Model file for the job. Use its own axes, mm. Face numbers are marked on the shaded views. A direction names the side the tool comes from. Give positions to 0.01 mm unless a question says otherwise; leave off trailing zeros. Order: outer loops, then holes, each group sorted by start corner. A loop starts at its lowest first (then second) coordinate and runs counter-clockwise, first axis right, second up. Notation, with made-up numbers: (-24.75, 48.5) - (0.25, 48.5) arc R14 cw to (0.25, 62.5) - close; hole circle Ø4 at (13.5, 47.5). An arc over 180 degrees is marked (long way). Return JSON: item names as keys, results as strings. Group by question number.
from build123d import *

# Parameters (mm, degrees)
F1_DEPTH = 2
F2_DEPTH = 19
F3_W     = 65
F3_H     = 2
F4_DEPTH = 25
F5_R     = 6
F6_DEPTH = 2.001


with BuildPart() as f1:
    # F0 (on Top) → F1 (new body)
    with BuildSketch(Plane.XY):
        Polygon((0, 32.5), (0, 17.5), (17.5, 17.5), (17.5, -17.5), (0, -17.5), (0, -32.5), (35, -32.5), (35, 0), (35, 32.5), align=None)
    extrude(amount=-F1_DEPTH)

    # F0 (on Top) → F2 (join)
    with BuildSketch(Plane.XY):
        Polygon((37, 32.5), (35, 32.5), (35, 0), (35, -32.5), (37, -32.5), align=None)
    extrude(amount=-F2_DEPTH)

    # F3 (on face) → F4 (join)
    with BuildSketch(Plane.YZ.offset(37)):
        with Locations((0, -18)):
            Rectangle(F3_W, F3_H)
    extrude(amount=F4_DEPTH)

    # F5 (on face) → F6 (cut, through all)
    with BuildSketch(Plane.XY.offset(-17)):
        with Locations((50, 0)):
            Circle(F5_R)
    extrude(amount=-F6_DEPTH, mode=Mode.SUBTRACT)

    # F7: F1 across face


with BuildPart() as f1_1:
    add(f1.part)
    add(f1.part.mirror(Plane(origin=(0, 25, -1), x_dir=(0, -1, 0), z_dir=(-1, 0, 0))))


solid = f1_1.part
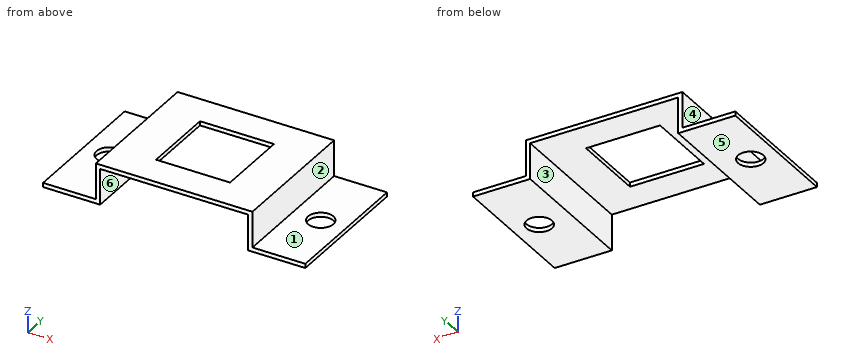
(1) Slice it at B-B (y = 13.5). Give the cut face in (x, z).
(2) Slice it at A-A (x = -50). Give the cut face in (y, z).
(3) 3-axis set-ups, long thin cutter, end or side, ignore diameter. For the marked faces 4, 5 and 6: which of +Z, -Z, +X, -X, +Y, -Y reach the whole face in a straight line?
(4) Pull direction X, two halves, no side cores. Call the marked faces 1, 2 and 3: released by +X, released by -X, zero draft, split by the parting line, or undercut.
(5) Drop flat-ended pins along their axis: pin 1 Ø14 at (x, y) = (50, 0) entering from +Z; pin 2 Ø2 at (y, z) = (-6, -1.5) entering from -X; pin 3 Ø5 at (y, z) = (-16, -7) entering from +X; pin 4 Ø10 at (x, y) = (-5.5, -19.5) entering from +Z. Give the stop position or say it passes through.
(6) Slice it at C-C (z = -9.5). Give the cut face in (x, y).
(7) Slice it at D-D (y = 0). Give the cut face in (x, z), and give its area (3 significant figures).
(8) Drill centre lines: L1, parallel to Y at x = 50, z = -17.9; L2, parallel to X at y = 11.5, z = -13.25; L3, parallel to Z at x = 33.5, y = -14. Where is each one in solid material? Low to high.
Result set:
{
 "1": {"outline": "(-62, -19) - (-35, -19) - (-35, -2) - (-17.5, -2) - (-17.5, 0) - (-37, 0) - (-37, -17) - (-62, -17) - close; (17.5, -2) - (35, -2) - (35, -19) - (62, -19) - (62, -17) - (37, -17) - (37, 0) - (17.5, 0) - close"},
 "2": {"outline": "(-32.5, -19) - (-6, -19) - (-6, -17) - (-32.5, -17) - close; (6, -19) - (32.5, -19) - (32.5, -17) - (6, -17) - close"},
 "3": {"face 4": "+Z, -X, +Y, -Y", "face 5": "-Z, +X, -X, +Y, -Y", "face 6": "-Z, +Y, -Y"},
 "4": {"face 1": "zero draft", "face 2": "released by +X", "face 3": "undercut"},
 "5": {"pin 1": "stops at z = -17", "pin 2": "stops at x = -37", "pin 3": "stops at x = 37", "pin 4": "stops at z = 0"},
 "6": {"outline": "(-37, -32.5) - (-35, -32.5) - (-35, 32.5) - (-37, 32.5) - close; (35, -32.5) - (37, -32.5) - (37, 32.5) - (35, 32.5) - close"},
 "7": {"outline": "(-62, -19) - (-56, -19) - (-56, -17) - (-62, -17) - close; (-44, -19) - (-35, -19) - (-35, -2) - (-17.5, -2) - (-17.5, 0) - (-37, 0) - (-37, -17) - (-44, -17) - close; (17.5, -2) - (35, -2) - (35, -19) - (44, -19) - (44, -17) - (37, -17) - (37, 0) - (17.5, 0) - close; (56, -19) - (62, -19) - (62, -17) - (56, -17) - close", "area": "198 mm²"},
 "8": {"L1": "y = -32.5 to -6, 6 to 32.5", "L2": "x = -37 to -35, 35 to 37", "L3": "z = -2 to 0"}
}
